Check sheet for the modelled part. Datum: model origin and axes. Units: mm. Face numbers are marked on the shaded views. A direction names the side the tool comes from. Give positions to 0.01 mm unless a question says otherwise; leave off trailing zeros. Write each loop counter-clockwise with the first axis right and the second up, starting at its lowest first coordinate (ties: lowest second). Pieces come first, ordered by that corner, then holes.
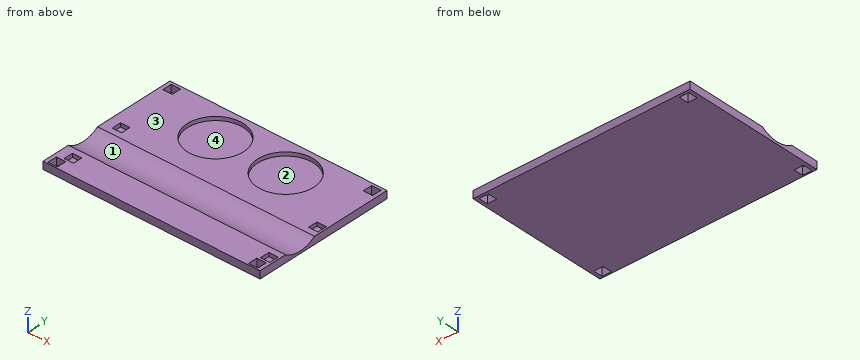
from build123d import *

# Parameters (mm, degrees)
SKETCH3_W           = 147.32
SKETCH3_H           = 96.52
BOSS_EXTRUDE1_DEPTH = 5.08
SKETCH4_R           = 19.05
SKETCH4_W           = 6.35
SKETCH4_H           = 6.35
CUT_EXTRUDE1_DEPTH  = 2.54
SKETCH6_W           = 6.35
SKETCH6_H           = 6.35
CUT_EXTRUDE3_DEPTH  = 7.62
SKETCH7_R           = 19.05
CUT_EXTRUDE4_DEPTH  = 171.45


with BuildPart() as part:
    # Sketch3 → Boss-Extrude1 (new body)
    with BuildSketch(Plane.XY):
        with Locations((85.663850978, -7.59744867)):
            Rectangle(SKETCH3_W, SKETCH3_H)
    extrude(amount=BOSS_EXTRUDE1_DEPTH)

    # Sketch4 → Cut-Extrude1 (cut)
    with BuildSketch(Plane.XY.offset(5.08)):
        with Locations((63.032517405, 18.070386575)):
            Circle(SKETCH4_R)
        with Locations((110.718650705, 18.070386575)):
            Circle(SKETCH4_R)
        with Locations((21.528850978, -43.79244867)):
            Rectangle(SKETCH4_W, SKETCH4_H)
        with Locations((154.878850978, -43.79244867)):
            Rectangle(SKETCH4_W, SKETCH4_H)
        with Locations((154.878850978, -7.21644867)):
            Rectangle(SKETCH4_W, SKETCH4_H)
        with Locations((21.528850978, -7.21644867)):
            Rectangle(SKETCH4_W, SKETCH4_H)
    extrude(amount=-CUT_EXTRUDE1_DEPTH, mode=Mode.SUBTRACT)

    # Sketch6 → Cut-Extrude3 (cut)
    with BuildSketch(Plane.XY):
        with Locations((17.679985474, -51.638260567)):
            Rectangle(SKETCH6_W, SKETCH6_H)
        with Locations((17.679985474, 35.579793927)):
            Rectangle(SKETCH6_W, SKETCH6_H)
        with Locations((153.766691322, 35.579793927)):
            Rectangle(SKETCH6_W, SKETCH6_H)
        with Locations((153.766691322, -51.638260567)):
            Rectangle(SKETCH6_W, SKETCH6_H)
    extrude(amount=CUT_EXTRUDE3_DEPTH, mode=Mode.SUBTRACT)

    # Sketch7 → Cut-Extrude4 (cut)
    with BuildSketch(Plane(origin=(0, 0, 0), x_dir=(0, 0, -1), z_dir=(1, 0, 0))):
        with Locations((-20.586973595, -25.47459189)):
            Circle(SKETCH7_R)
    extrude(amount=CUT_EXTRUDE4_DEPTH, mode=Mode.SUBTRACT)


solid = part.part
1) Sectioned sample at D-D on x = 47. Record the boundary of the cut face in (y, z), then the cut area to 3 significant figures.
2) Sectioned sample at A-A on z = 3.95. Give the number of separate pieces and of enclosed holes in the cut face, then the cut area to 3 significant figures.
3) Scan lines: L1, parallel to X at y = 17, z = 4.6; L2, parallel to X at y = 34, z = 1.3; L3, parallel to Y at x = 107, z = 4.35. Record each from-to range of solid material in increasing order.
4) Access from +Z, -Z, +X, -X, +Y, -Y to the whole of each face (thin tool, end or side, straight path). Record for the marked faces 3 and 4.
5) Sectioned sample at C-C on y = 24.5. Record the boundary of the cut face in (x, z), then the cut area to 3 significant figures.
6) Sectioned sample at B-B on x = 136. Record the boundary of the cut face in (y, z), then the cut area to 3 significant figures.
7) Gauge pin test, flat end, axial feed: pin 1 (3 mm diameter, centred on x = 156, y = -7, fed in from +Z). Record the tip position at first contact, or that the pin passes through.
8) Draft check along X on the marked faces 1 and 2. Enter one of: +X half, -X half, draft (parallel to the pull), parting line (faces both ways), or undercut.
Answers below:
1. outline: (-55.86, 0) - (40.66, 0) - (40.66, 5.08) - (28.36, 5.08) - (28.36, 2.54) - (7.78, 2.54) - (7.78, 5.08) - (-14.41, 5.08) arc R19.05 cw to (-36.54, 5.08) - (-55.86, 5.08) - close
1. area: 385 mm2
2. separate pieces: 2
2. enclosed holes: 10
2. area: 8,880 mm2
3. L1: x = 12 to 44.01, 82.05 to 91.7, 129.74 to 159.32
3. L2: x = 12 to 14.5, 20.85 to 150.59, 156.94 to 159.32
3. L3: y = -55.86 to -35.44, -15.51 to -0.61, 36.75 to 40.66
4. face 3: +Z, +X, -X, +Y, -Y
4. face 4: +Z
5. outline: (12, 0) - (159.32, 0) - (159.32, 5.08) - (128.65, 5.08) - (128.65, 2.54) - (92.79, 2.54) - (92.79, 5.08) - (80.96, 5.08) - (80.96, 2.54) - (45.1, 2.54) - (45.1, 5.08) - (12, 5.08) - close
5. area: 566 mm2
6. outline: (-55.86, 0) - (40.66, 0) - (40.66, 5.08) - (-14.41, 5.08) arc R19.05 cw to (-36.54, 5.08) - (-55.86, 5.08) - close
6. area: 437 mm2
7. pin 1: stops at z = 2.54
8. face 1: draft
8. face 2: undercut
